Design review of the part built by this model. Coordinates are the model's own, in mm. Give positions to 0.01 mm unless a question says otherwise; leave off trailing zeros. Write each loop counter-clockwise with the first axis right and the second up, starting at its lowest first coordinate (ties: lowest second). Pieces come first, ordered by that corner, then holes. Notation, with made-up numbers: (17.25, 71) -> (73.25, 71) arc R24 cw to (73.25, 105) -> close; hole circle Ø5 at (39.5, 75.5). An arc over 180 degrees is marked (long way). Answer as a JSON object with one key per item and string values.
```python
from build123d import *

# Parameters (mm, degrees)
F0_R       = 6.5146341495
F1_DEPTH   = 7
F2_R       = 150
F3_SIZE2   = 3.4641016151
F3_SIZE    = 2
F3_2_SIZE2 = 3.4641016151
F3_2_SIZE  = 2


with BuildPart() as f1:
    # F0 (on Top) → F1 (new body)
    with BuildSketch(Plane.XY):
        with BuildLine():
            ThreePointArc((20.3305371016, 10.8474336629), (18.8276716907, 14.0034842548), (16.9554240496, 16.9554240496))
            ThreePointArc((16.9554240496, 16.9554240496), (14.0082290327, 18.8250492727), (10.8574857337, 20.3264731323))
            ThreePointArc((10.8574857337, 20.3264731323), (10.8576641201, 20.2905395913), (10.8577235824, 20.2546056568))
            ThreePointArc((10.8577235824, 20.2546056568), (-0.0359339345, 9.3969415367), (-10.8574857337, 20.3264731323))
            ThreePointArc((-10.8574857337, 20.3264731323), (-14.0082290327, 18.8250492727), (-16.9554240496, 16.9554240496))
            ThreePointArc((-16.9554240496, 16.9554240496), (-18.8254179031, 14.0075621913), (-20.3270445442, 10.8560730228))
            ThreePointArc((-20.3270445442, 10.8560730228), (-12.5273872935, 7.7442134548), (-9.280006631, 0))
            ThreePointArc((-9.280006631, 0), (-12.5273872935, -7.7442134548), (-20.3270445442, -10.8560730228))
            ThreePointArc((-20.3270445442, -10.8560730228), (-18.8254179031, -14.0075621913), (-16.9554240496, -16.9554240496))
            ThreePointArc((-16.9554240496, -16.9554240496), (-14.1911797406, -18.7230451047), (-11.2446974396, -20.1665730208))
            ThreePointArc((-11.2446974396, -20.1665730208), (-0.1727046676, -8.5725301074), (11.25, -19.8212043892))
            ThreePointArc((11.25, -19.8212043892), (11.2486742818, -19.9939090568), (11.2446974396, -20.1665730208))
            ThreePointArc((11.2446974396, -20.1665730208), (14.1911797406, -18.7230451047), (16.9554240496, -16.9554240496))
            ThreePointArc((16.9554240496, -16.9554240496), (18.8276716907, -14.0034842548), (20.3305371016, -10.8474336629))
            ThreePointArc((20.3305371016, -10.8474336629), (9.0002203311, 0), (20.3305371016, 10.8474336629))
        make_face()
        Circle(F0_R, mode=Mode.SUBTRACT)
        with BuildLine():
            ThreePointArc((-16.9554240496, 16.9554240496), (-20.5343741855, 13.8978501036), (-23.5705866136, 10.300760085))
            ThreePointArc((-23.5705866136, 10.300760085), (-21.9699756434, 10.7020109361), (-20.3270445442, 10.8560730228))
            ThreePointArc((-20.3270445442, 10.8560730228), (-18.8254179031, 14.0075621913), (-16.9554240496, 16.9554240496))
        make_face()
        with BuildLine():
            ThreePointArc((-6.4970776314, 28.9539242303), (-15.4163775625, 27.5515698423), (-23.470058199, 23.470058199))
            ThreePointArc((-23.470058199, 23.470058199), (-27.5758715938, 15.3408078623), (-28.9533926969, 6.3383165249))
            ThreePointArc((-28.9533926969, 6.3383165249), (-26.5744835451, 8.7440475719), (-23.5705866136, 10.300760085))
            ThreePointArc((-23.5705866136, 10.300760085), (-20.5343741855, 13.8978501036), (-16.9554240496, 16.9554240496))
            ThreePointArc((-16.9554240496, 16.9554240496), (-13.9194172815, 20.5129124867), (-10.3502609953, 23.5351938238))
            ThreePointArc((-10.3502609953, 23.5351938238), (-8.8486645605, 26.5467672001), (-6.4970776314, 28.9539242303))
        make_face()
        with BuildLine():
            ThreePointArc((-10.8574857337, 20.3264731323), (-10.7245560491, 21.9499106272), (-10.3502609953, 23.5351938238))
            ThreePointArc((-10.3502609953, 23.5351938238), (-13.9194172815, 20.5129124867), (-16.9554240496, 16.9554240496))
            ThreePointArc((-16.9554240496, 16.9554240496), (-14.0082290327, 18.8250492727), (-10.8574857337, 20.3264731323))
        make_face()
        with BuildLine():
            ThreePointArc((-28.9533926969, -6.3383165249), (-27.5758715938, -15.3408078623), (-23.470058199, -23.470058199))
            ThreePointArc((-23.470058199, -23.470058199), (-15.4507716917, -27.5404335913), (-6.5693817436, -28.9538777933))
            ThreePointArc((-6.5693817436, -28.9538777933), (-9.0925043483, -26.4460715332), (-10.7064490846, -23.2758314312))
            ThreePointArc((-10.7064490846, -23.2758314312), (-14.0749053099, -20.3568391805), (-16.9554240496, -16.9554240496))
            ThreePointArc((-16.9554240496, -16.9554240496), (-20.5343741855, -13.8978501036), (-23.5705866136, -10.300760085))
            ThreePointArc((-23.5705866136, -10.300760085), (-26.5744835451, -8.7440475719), (-28.9533926969, -6.3383165249))
        make_face()
        with BuildLine():
            ThreePointArc((-6.5693817436, -28.9538777933), (-15.4507716917, -27.5404335913), (-23.470058199, -23.470058199))
            ThreePointArc((-23.470058199, -23.470058199), (0, -35.4685637026), (23.470058199, -23.470058199))
            ThreePointArc((23.470058199, -23.470058199), (15.4507716917, -27.5404335913), (6.5693817436, -28.9538777933))
            ThreePointArc((6.5693817436, -28.9538777933), (0, -31.0712043892), (-6.5693817436, -28.9538777933))
        make_face()
        with BuildLine():
            ThreePointArc((-28.9533926969, 6.3383165249), (-27.5758715938, 15.3408078623), (-23.470058199, 23.470058199))
            ThreePointArc((-23.470058199, 23.470058199), (-35.4685637026, 0), (-23.470058199, -23.470058199))
            ThreePointArc((-23.470058199, -23.470058199), (-27.5758715938, -15.3408078623), (-28.9533926969, -6.3383165249))
            ThreePointArc((-28.9533926969, -6.3383165249), (-30.9954537959, 0), (-28.9533926969, 6.3383165249))
        make_face()
        with BuildLine():
            ThreePointArc((6.4970776314, 28.9539242303), (15.4163775625, 27.5515698423), (23.470058199, 23.470058199))
            ThreePointArc((23.470058199, 23.470058199), (0, 35.4685637026), (-23.470058199, 23.470058199))
            ThreePointArc((-23.470058199, 23.470058199), (-15.4163775625, 27.5515698423), (-6.4970776314, 28.9539242303))
            ThreePointArc((-6.4970776314, 28.9539242303), (0, 31.1123292392), (6.4970776314, 28.9539242303))
        make_face()
        with BuildLine():
            ThreePointArc((28.9481833992, 5.9378200954), (28.952492979, 6.2262128121), (28.9539295531, 6.5146341495))
            ThreePointArc((28.9539295531, 6.5146341495), (27.5488697433, 15.424730245), (23.470058199, 23.470058199))
            ThreePointArc((23.470058199, 23.470058199), (15.4163775625, 27.5515698423), (6.4970776314, 28.9539242303))
            ThreePointArc((6.4970776314, 28.9539242303), (8.8486645605, 26.5467672001), (10.3502609953, 23.5351938238))
            ThreePointArc((10.3502609953, 23.5351938238), (13.9194172815, 20.5129124867), (16.9554240496, 16.9554240496))
            ThreePointArc((16.9554240496, 16.9554240496), (20.591369411, 13.8403539947), (23.6642529801, 10.1686858877))
            ThreePointArc((23.6642529801, 10.1686858877), (26.6443492565, 8.4755450511), (28.9481833992, 5.9378200954))
        make_face()
        with BuildLine():
            ThreePointArc((16.9554240496, 16.9554240496), (13.9194172815, 20.5129124867), (10.3502609953, 23.5351938238))
            ThreePointArc((10.3502609953, 23.5351938238), (10.7245560491, 21.9499106272), (10.8574857337, 20.3264731323))
            ThreePointArc((10.8574857337, 20.3264731323), (14.0082290327, 18.8250492727), (16.9554240496, 16.9554240496))
        make_face()
        with BuildLine():
            ThreePointArc((20.3305371016, 10.8474336629), (22.0241446803, 10.6394424492), (23.6642529801, 10.1686858877))
            ThreePointArc((23.6642529801, 10.1686858877), (20.591369411, 13.8403539947), (16.9554240496, 16.9554240496))
            ThreePointArc((16.9554240496, 16.9554240496), (18.8276716907, 14.0034842548), (20.3305371016, 10.8474336629))
        make_face()
        with BuildLine():
            ThreePointArc((23.470058199, 23.470058199), (27.5488697433, 15.424730245), (28.9539295531, 6.5146341495))
            ThreePointArc((28.9539295531, 6.5146341495), (28.952492979, 6.2262128121), (28.9481833992, 5.9378200954))
            ThreePointArc((28.9481833992, 5.9378200954), (30.2644195183, 3.0976486049), (30.7156674959, 0))
            ThreePointArc((30.7156674959, 0), (30.2644195183, -3.0976486049), (28.9481833992, -5.9378200954))
            ThreePointArc((28.9481833992, -5.9378200954), (28.952492979, -6.2262128121), (28.9539295531, -6.5146341495))
            ThreePointArc((28.9539295531, -6.5146341495), (27.5488697433, -15.424730245), (23.470058199, -23.470058199))
            ThreePointArc((23.470058199, -23.470058199), (32.2950161292, -13.1796032393), (35.4685637026, 0))
            ThreePointArc((35.4685637026, 0), (32.2950161292, 13.1796032393), (23.470058199, 23.470058199))
        make_face()
        with BuildLine():
            ThreePointArc((16.9554240496, -16.9554240496), (20.591369411, -13.8403539947), (23.6642529801, -10.1686858877))
            ThreePointArc((23.6642529801, -10.1686858877), (22.0241446803, -10.6394424492), (20.3305371016, -10.8474336629))
            ThreePointArc((20.3305371016, -10.8474336629), (18.8276716907, -14.0034842548), (16.9554240496, -16.9554240496))
        make_face()
        with BuildLine():
            ThreePointArc((-16.9554240496, -16.9554240496), (-14.0749053099, -20.3568391805), (-10.7064490846, -23.2758314312))
            ThreePointArc((-10.7064490846, -23.2758314312), (-11.0851287948, -21.7401675475), (-11.2446974396, -20.1665730208))
            ThreePointArc((-11.2446974396, -20.1665730208), (-14.1911797406, -18.7230451047), (-16.9554240496, -16.9554240496))
        make_face()
        with BuildLine():
            ThreePointArc((-20.3270445442, -10.8560730228), (-21.9699756434, -10.7020109361), (-23.5705866136, -10.300760085))
            ThreePointArc((-23.5705866136, -10.300760085), (-20.5343741855, -13.8978501036), (-16.9554240496, -16.9554240496))
            ThreePointArc((-16.9554240496, -16.9554240496), (-18.8254179031, -14.0075621913), (-20.3270445442, -10.8560730228))
        make_face()
        with BuildLine():
            ThreePointArc((6.5693817436, -28.9538777933), (15.4507716917, -27.5404335913), (23.470058199, -23.470058199))
            ThreePointArc((23.470058199, -23.470058199), (27.5488697433, -15.424730245), (28.9539295531, -6.5146341495))
            ThreePointArc((28.9539295531, -6.5146341495), (28.952492979, -6.2262128121), (28.9481833992, -5.9378200954))
            ThreePointArc((28.9481833992, -5.9378200954), (26.6443492565, -8.4755450511), (23.6642529801, -10.1686858877))
            ThreePointArc((23.6642529801, -10.1686858877), (20.591369411, -13.8403539947), (16.9554240496, -16.9554240496))
            ThreePointArc((16.9554240496, -16.9554240496), (14.0749053099, -20.3568391805), (10.7064490846, -23.2758314312))
            ThreePointArc((10.7064490846, -23.2758314312), (9.0925043483, -26.4460715332), (6.5693817436, -28.9538777933))
        make_face()
        with BuildLine():
            ThreePointArc((10.7064490846, -23.2758314312), (14.0749053099, -20.3568391805), (16.9554240496, -16.9554240496))
            ThreePointArc((16.9554240496, -16.9554240496), (14.1911797406, -18.7230451047), (11.2446974396, -20.1665730208))
            ThreePointArc((11.2446974396, -20.1665730208), (11.0851287948, -21.7401675475), (10.7064490846, -23.2758314312))
        make_face()
    extrude(amount=F1_DEPTH)

    # F2
    f2_edges = [f1.edges().sort_by_distance(p)[0] for p in [
        (23.470058, -23.470058, 3.5),
        (23.470058, 23.470058, 3.5),
        (-23.470058, 23.470058, 3.5),
        (-23.470058, -23.470058, 3.5),
    ]]
    fillet(f2_edges, radius=F2_R)

    # F3
    f3_edges = [f1.edges().sort_by_distance(p)[0] for p in [
        (-35.468564, 0, 7),
    ]]
    f3_side = f1.faces().sort_by_distance((0, -34.465361, 7))[0]
    chamfer(f3_edges, length=F3_SIZE, length2=F3_SIZE2, reference=f3_side)

    # F3#2
    f3_2_edges = [f1.edges().sort_by_distance(p)[0] for p in [
        (-35.468564, 0, 0),
    ]]
    f3_2_side = f1.faces().sort_by_distance((0, -34.465361, 0))[0]
    chamfer(f3_2_edges, length=F3_2_SIZE, length2=F3_2_SIZE2, reference=f3_2_side)


solid = f1.part
```
(1) We need section A-A, the plane x = 0. State the section outline as (y, z) points.
Here are the results:
{"outline": "(-35.47, 3.46) -> (-33.47, 0) -> (-31.07, 0) -> (-31.07, 7) -> (-33.47, 7) -> (-35.47, 3.54) -> close; (-8.57, 0) -> (-6.51, 0) -> (-6.51, 7) -> (-8.57, 7) -> close; (6.51, 0) -> (9.4, 0) -> (9.4, 7) -> (6.51, 7) -> close; (31.11, 0) -> (33.47, 0) -> (35.47, 3.46) -> (35.47, 3.54) -> (33.47, 7) -> (31.11, 7) -> close"}
(2) We need section B-B, the plane z = 2. Give the number of separate pieces and of enclosed holes in the cut face, then the cut area to 3 significant figures.
Here are the results:
{"separate pieces": "1", "enclosed holes": "5", "area": "1,960 mm²"}
(3) Clearance check with flat-ended pins moving along their axes: pin 1 (2 mm diameter, centred on y = -23, z = 4, fed in from +X); pin 2 (4 mm diameter, centred on y = -9.5, z = 3, fed in from +X); pin 3 (2 mm diameter, centred on y = 5, z = 3.5, fed in from -X). State where each tip first meets the part, or that it passes through.
Here are the results:
{"pin 1": "stops at x = 25.29", "pin 2": "stops at x = 34.47", "pin 3": "stops at x = -35.19"}
(4) The part is to be moulded in two halves that separate along X. For faces 1 (the conical face through (-0.31, -33.814, 0.602)), 2 (the flat face through (0, -7, 7)), 3 (the cylindrical face through (-1.41, -6.36, 3.45)), 4 (the conical face through (-33.814, 0.31, 0.602)), say which applies: +X half, -X half, draft (parallel to the pull), parting line (faces both ways), or undercut.
Here are the results:
{"face 1": "parting line", "face 2": "draft", "face 3": "undercut", "face 4": "-X half"}
(5) For line 1 along X through (y, z) = (-4, 4.5); line 2 along Y through (x, z) = (7, 3.25); line 3 along X through (y, z) = (-8.5, 1.5), list the stretches that pass through material, from the lowest coordinate up.
Here are the results:
{"line 1": "x = -34.63 to -30.23, -10.04 to -5.14, 5.14 to 9.76, 29.95 to 34.63", "line 2": "y = -34.48 to -28.63, -11.01 to 11.95, 28.55 to 34.48", "line 3": "x = -33 to -26.89, -13.38 to 13.1, 26.61 to 33"}
